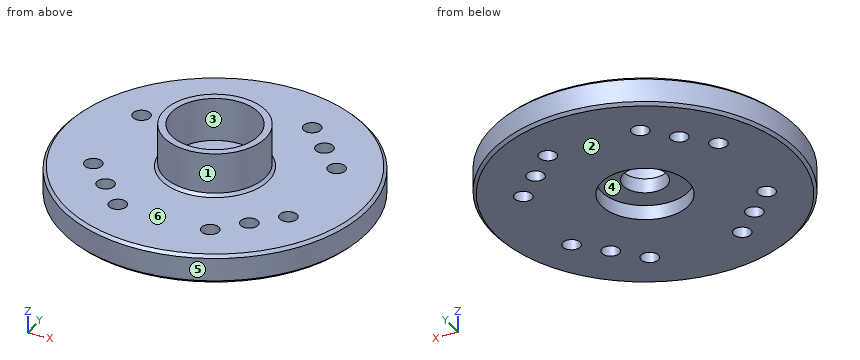
from build123d import *

# Parameters (mm, degrees)
SKETCH_1_R          = 10.5
SKETCH_1_R_2        = 1.5
EXTRUDE_1_DEPTH     = 2
SKETCH_2_R          = 3.5
SKETCH_2_R_2        = 3
EXTRUDE_2_DEPTH     = 3
SKETCH_3_R          = 3
CUT_EXTRUDE_1_DEPTH = 1
SKETCH_4_R          = 0.6
CUT_EXTRUDE_2_DEPTH = 2
CHAMFER_1_SIZE      = 0.2


with BuildPart() as part:
    # 草图1 → 凸台-拉伸1 (new body)
    with BuildSketch(Plane.XY):
        Circle(SKETCH_1_R)
        Circle(SKETCH_1_R_2, mode=Mode.SUBTRACT)
    extrude(amount=EXTRUDE_1_DEPTH)

    # 草图2 → 凸台-拉伸2 (add)
    with BuildSketch(Plane.XY.offset(2)):
        Circle(SKETCH_2_R)
        Circle(SKETCH_2_R_2, mode=Mode.SUBTRACT)
    extrude(amount=EXTRUDE_2_DEPTH)

    # 草图3 → 切除-拉伸1 (cut)
    with BuildSketch(Plane(origin=(0, 0, 0), x_dir=(-1, 0, 0), z_dir=(0, 0, -1))):
        with Locations(Location((0, 0, 0), (0, 0, 180))):
            Circle(SKETCH_3_R)
    extrude(amount=-CUT_EXTRUDE_1_DEPTH, mode=Mode.SUBTRACT)

    # 草图4 → 切除-拉伸2 (cut)
    with BuildSketch(Plane.XY.offset(2)):
        with Locations((-4.949747468, 4.949747468)):
            Circle(SKETCH_4_R)
        with Locations((4.949747468, 4.949747468)):
            Circle(SKETCH_4_R)
        with Locations((-4.949747468, -4.949747468)):
            Circle(SKETCH_4_R)
        with Locations((4.949747468, -4.949747468)):
            Circle(SKETCH_4_R)
        with Locations((-3.181980515, 6.717514421)):
            Circle(SKETCH_4_R)
        with Locations(Location((-6.717514421, 3.181980515, 0), (0, 0, 180))):
            Circle(SKETCH_4_R)
        with Locations((6.717514421, 3.181980515)):
            Circle(SKETCH_4_R)
        with Locations(Location((3.181980515, 6.717514421, 0), (0, 0, 180))):
            Circle(SKETCH_4_R)
        with Locations((3.181980515, -6.717514421)):
            Circle(SKETCH_4_R)
        with Locations(Location((6.717514421, -3.181980515, 0), (0, 0, 180))):
            Circle(SKETCH_4_R)
        with Locations((-6.717514421, -3.181980515)):
            Circle(SKETCH_4_R)
        with Locations(Location((-3.181980515, -6.717514421, 0), (0, 0, 180))):
            Circle(SKETCH_4_R)
    extrude(amount=-CUT_EXTRUDE_2_DEPTH, mode=Mode.SUBTRACT)

    # 倒角1
    chamfer_1_edges = [part.edges().sort_by_distance(p)[0] for p in [
        (-3.5, 0, 2),
        (-10.5, 0, 0),
        (-10.5, 0, 2),
    ]]
    chamfer(chamfer_1_edges, length=CHAMFER_1_SIZE)


solid = part.part
Geometry: final body of the model. Coordinates: model frame, mm. Face numbers are marked on the shaded views. A direction names the side the tool comes from. Coordinates: 2 decimals unless noted, no trailing zeros. Order: outer loops, then holes, each group sorted by start corner. A loop starts at its lowest first (then second) coordinate and runs counter-clockwise, first axis right, second up.
1) Section C-C (z = 0.75). Give the number of separate pieces and of enclosed holes in the cut face, then the cut area to 3 significant figures.
Result sheet:
separate pieces: 1
enclosed holes: 13
area: 305 mm2
2) Ray query, probe 1 along Z at (x, y) = (-7, -5.5); probe 2 along X at (y, z) = (3.25, 1.25); probe 3 along X at (y, z) = (2, 1.4). Return the intervals inside material, ascending.
Result sheet:
probe 1: z = 0 to 2
probe 2: x = -9.98 to -7.31, -6.12 to 6.12, 7.31 to 9.98
probe 3: x = -10.31 to 10.31
3) Section A-A (y = 0). Return loops of the section in (x, z), then the cut area to 3 significant figures.
Result sheet:
outline: (-10.5, 0.2) - (-10.3, 0) - (-3, 0) - (-3, 1) - (-1.5, 1) - (-1.5, 2) - (-3, 2) - (-3, 5) - (-3.5, 5) - (-3.5, 2.2) - (-3.7, 2) - (-10.3, 2) - (-10.5, 1.8) - close; (1.5, 1) - (3, 1) - (3, 0) - (10.3, 0) - (10.5, 0.2) - (10.5, 1.8) - (10.3, 2) - (3.7, 2) - (3.5, 2.2) - (3.5, 5) - (3, 5) - (3, 2) - (1.5, 2) - close
area: 36.0 mm2
4) First-contact query: P1, Ø1.6, axis at x = -3.18, y = 6.72, coming from the +Z side; P2, Ø1.5, axis at x = 7, z = 2.5, coming from the +Y side; P3, Ø1.8, axis at x = 1.5, y = 1, coming from the -Z side. Flat tips, straight axial feed; report the tip coordinate or a pass-through.
Result sheet:
P1: stops at z = 2
P2: stops at y = 8.08
P3: stops at z = 1
5) Draft query along X for the marked faces 3, 4, 5 and 6. Return one class per face: released by +X, released by -X, zero draft, split by the parting line, or undercut.
Result sheet:
face 3: undercut
face 4: undercut
face 5: split by the parting line
face 6: zero draft
6) Set-up query: the marked faces 1 and 2. Return all of +Z, -Z, +X, -X, +Y, -Y with unobstructed straight access to the full face (end or side cutting, diameter ignored); none if empty.
Result sheet:
face 1: +Z
face 2: -Z, +X, -X, +Y, -Y
